Read the model definition and answer for the solid it produces. Units are mm, in the model's axes. A direction names the side the tool comes from. Round coordinates to 2 decimals unless told otherwise and drop trailing zeros. Write each loop counter-clockwise with the first axis right and the second up, starting at its lowest first coordinate (ties: lowest second). Pieces come first, ordered by that corner, then holes.
Autodesk Inventor part; units mm, degrees
ref_plane "Work Plane1" through (-8.075, -22.5, -2.8) normal (0, 0, 1) x (1, 0, 0)
ref_plane "YZ Plane" through (0, 0, 0) normal (1, 0, 0) x (0, 1, 0)
ref_plane "XZ Plane" through (0, 0, 0) normal (0, 1, 0) x (-1, 0, 0)
sketch "sk_main" plane through (0, 0, 0) normal (0, 0, 1) x (1, 0, 0)
  arc A0 (-6.075, -0.5) -> (-8.075, -2.5) centre (-6.075, -2.5) ccw
  line L0 (-8.075, -20.5) -> (-8.075, -2.5)
  arc A1 (-8.075, -20.5) -> (-6.075, -22.5) centre (-6.075, -20.5) ccw
  line L1 (-6.075, -22.5) -> (6.075, -22.5)
  arc A2 (6.075, -22.5) -> (8.075, -20.5) centre (6.075, -20.5) ccw
  line L2 (8.075, -2.5) -> (8.075, -20.5)
  arc A3 (8.075, -2.5) -> (6.075, -0.5) centre (6.075, -2.5) ccw
  line L3 (-6.075, -0.5) -> (6.075, -0.5)
  circle A4 centre (-5, -2.5) radius 1
  circle A5 centre (0, -20) radius 1
  circle A6 centre (-5.075, -11) radius 1
  circle A7 centre (5.075, -11) radius 1
  circle A8 centre (5, -2.5) radius 1
  circle A9 centre (0, -11) radius 3.4
  circle A10 centre (0, -20) radius 2.75
  line L4 (-2, -21.8875) -> (-2, -22.5)
  line L5 (2, -21.8875) -> (2, -22.5)
  line L6 (0, 4.5828) -> (0, -27.4971)
  circle A11 centre (0, -11) radius 5.25
  arc A12 (-5.1545, -10.0032) -> (-5.1545, -11.9968) centre (-5.075, -11) ccw
  arc A13 (5.1545, -11.9968) -> (5.1545, -10.0032) centre (5.075, -11) ccw
  point P0 (0, 0)
  dimension "d1" = 5.5
  dimension "d2" = 4
  dimension "d3" = 10.5
extrude "ext_main" add sketch "sk_main" along normal blind 4 contours L3 L6 A11 A6 A10 L4 L1 A1 L0 A0 | L3 A3 L2 A2 L1 L5 A10 L6 A11 A7 | A7 A11 | A11 A6 | L4 A10 L1 | A10 L6 A5 L1 | L6 A5 A10 L1 | L1 A10 L5 picked at (5.5112, -11.1934) picked at (-5.5179, -11)
sketch "Sketch2" plane through (0, 0, 0) normal (0, 0, 1) x (1, 0, 0)
  line L0 (-6.075, -0.5) -> (6.075, -0.5)
  arc A0 (-6.075, -0.5) -> (-8.075, -2.5) centre (-6.075, -2.5) ccw
  line L1 (-8.075, -20.5) -> (-8.075, -2.5)
  arc A1 (8.075, -2.5) -> (6.075, -0.5) centre (6.075, -2.5) ccw
  line L2 (8.075, -2.5) -> (8.075, -20.5)
  circle A2 centre (5, -2.5) radius 1
  circle A3 centre (-5, -2.5) radius 1
  circle A4 centre (0, -11) radius 3.4
  circle A5 centre (0, -11) radius 8.25
  line L3 (-4.0318, -2.75) -> (4.0318, -2.75)
  line L4 (-5.5309, -3.3474) -> (-8.075, -7.408)
  circle A6 centre (0, -11) radius 8.75 construction
  line L5 (5.5309, -3.3474) -> (8.075, -7.408)
  line L6 (0, 4.1) -> (0, -24.6)
  arc A7 (-4.0318, -2.75) -> (-5.5309, -3.3474) centre (-5, -2.5) ccw
  arc A8 (5.5309, -3.3474) -> (4.0318, -2.75) centre (5, -2.5) ccw
  line L7 (6.5663, -5) -> (8.075, -5)
  line L8 (-6.5663, -5) -> (-8.075, -5)
  point P0 (0, 0)
  dimension "d6" = 16.5
  dimension "d7" = 0.5
  dimension "d8" = 4.5
ref_plane "Work Plane1" through (-8.075, -22.5, -2.8) normal (0, 0, 1) x (1, 0, 0)
extrude "ext_base" add sketch "Sketch2" against normal up to surface (2.8 mm away) contours L0 L6 L3 A3 L4 L8 L1 A0 | L0 A1 L2 L7 L5 A2 L3 L6
sketch "Sketch4" plane through (0, 0, 0) normal (0, 0, -1) x (-1, 0, 0)
  line L0 (6.075, -22.5) -> (-6.075, -22.5)
  circle A0 centre (0, -20) radius 1
  circle A1 centre (0, -20) radius 2.75
  line L1 (0, -27.4971) -> (0, 4.5828)
  line L2 (-2, -21.8875) -> (-2, -22.5)
  line L3 (2, -21.8875) -> (2, -22.5)
  point P0 (0, 0)
  dimension "d13" = 5.5
  dimension "d14" = 4
extrude "ext_cut_gearhousing" cut sketch "Sketch4" against normal blind 1.2 contours L0 A1 L3 | L0 L1 A0 A1 | L0 A1 L1 A0 | L0 L2 A1
sketch "Sketch3" plane through (0, 0, 4) normal (0, 0, 1) x (1, 0, 0)
  circle A0 centre (0, -20) radius 1
  point P0 (0, 0)
extrude "ext_dowelfill" add sketch "Sketch3" against normal blind 2
properties part number "linact_palm_front"
Q1. Section B-B (z = 3.5) is taken. Determine the outline of the cut face in (x, y) (3 decimals), then the cut area to 3 significant figures.
Verdict:
outline: (-8.075, -20.5) arc R2 ccw to (-6.075, -22.5) - (6.075, -22.5) arc R2 ccw to (8.075, -20.5) - (8.075, -2.5) arc R2 ccw to (6.075, -0.5) - (-6.075, -0.5) arc R2 ccw to (-8.075, -2.5) - close; hole circle Ø2 at (-5, -2.5); hole circle Ø10.5 at (0, -11); hole circle Ø2 at (5, -2.5)
area: 259 mm2
Q2. Straight lines are drawn through the part: probe 1 along X at (y, z) = (-2.5, 0.75) (3 decimals); probe 2 along Y at (x, z) = (0, 1.45); probe 3 along Y at (x, z) = (0, 0.45). For each, find the intervals that lie inside material, in ascending order.
Verdict:
probe 1: x = -8.075 to -6, -4 to 4, 6 to 8.075
probe 2: y = -22.5 to -21, -19 to -16.25, -5.75 to -0.5
probe 3: y = -17.25 to -16.25, -5.75 to -0.5
Q3. Section D-D (x = 0.5) is taken. Determine the outline of the cut face in (y, z), then the cut area to 3 significant figures.
Verdict:
outline: (-22.5, 1.2) - (-20.87, 1.2) - (-20.87, 2) - (-19.13, 2) - (-19.13, 1.2) - (-17.3, 1.2) - (-17.3, 0) - (-16.23, 0) - (-16.23, 4) - (-22.5, 4) - close; (-5.77, 0) - (-2.75, 0) - (-2.75, -2.8) - (-0.5, -2.8) - (-0.5, 4) - (-5.77, 4) - close
area: 44.9 mm2
Q4. Flat-ended cylindrical pins translate along their axes: pin 1 Ø2 at (x, y) = (-4.5, -15.5) entering from -Z; pin 2 Ø0.8 at (x, z) = (7.5, -1) entering from -Y; pin 3 Ø3.5 at (x, y) = (0, -20) entering from -Z. Find the tip coordinate at first contact, or state that the pin passes through.
Verdict:
pin 1: stops at z = 0
pin 2: stops at y = -5
pin 3: stops at z = 1.2
Q5. Which of the six approach directions +Z, -Z, +X, -X, +Y, -Y give full straight-line access (tool end or side, diameter ignored) to faces 4 (the cylindrical face through (7.474, -1.07, 0.552)), 5 (the flat face through (0, -17, 0)), 6 (the flat face through (0, -0.5, 1)), 7 (the flat face through (7, -5, -1)), 8 (the cylindrical face through (-0.217, -19.024, 1.594))?
Verdict:
face 4: +Z, -Z, +X, +Y
face 5: -Z, -Y
face 6: +Z, -Z, +X, -X, +Y
face 7: -Z, +X, -X, -Y
face 8: -Z
Q6. Determine the mould class of faces 1 (the flat face through (-7, -5, -1)), 2 (the cylindrical face through (5.46, -1.61, 0.55)), 3 (the flat face through (8.075, -11, 2)) for opening direction Y: pulls with the +Y half, pulls with the -Y half, needs draft (parallel to the pull), parting line crosses it, or undercut.
Verdict:
face 1: pulls with the -Y half
face 2: undercut
face 3: needs draft
Q7. Section C-C (y = -11) is taken. Determine the outline of the cut face in (x, z) (3 decimals), then the cut area to 3 significant figures.
Verdict:
outline: (-8.075, 0) - (-5.25, 0) - (-5.25, 4) - (-8.075, 4) - close; (5.25, 0) - (8.075, 0) - (8.075, 4) - (5.25, 4) - close
area: 22.6 mm2
Q8. Section A-A (y = -20) is taken. Determine the outline of the cut face in (x, z) (3 decimals), then the cut area to 3 significant figures.
Verdict:
outline: (-8.075, 0) - (-2.75, 0) - (-2.75, 1.2) - (-1, 1.2) - (-1, 2) - (1, 2) - (1, 1.2) - (2.75, 1.2) - (2.75, 0) - (8.075, 0) - (8.075, 4) - (-8.075, 4) - close
area: 56.4 mm2
